For this review, take the finished solid that the model builds, in its own axes (mm). A direction names the side the tool comes from. Round coordinates to 2 decimals unless told otherwise and drop trailing zeros. Write each loop counter-clockwise with the first axis right and the second up, starting at its lowest first coordinate (ties: lowest second). Pieces come first, ordered by that corner, then holes. Notation, with made-up numbers: (3.25, -34.75) -> (45.25, -34.75) arc R29 cw to (45.25, 2.25) -> close; hole circle Ø5 at (-10.5, 14). An arc over 180 degrees is marked (long way). Answer in a Markdown table with one row per item.
Autodesk Inventor part; units mm, degrees
ref_plane "YZ Plane" through (0, 0, 0) normal (1, 0, 0) x (0, 1, 0)
ref_plane "XZ Plane" through (0, 0, 0) normal (0, 1, 0) x (-1, 0, 0)
ref_plane "XY Plane" through (0, 0, 0) normal (0, 0, 1) x (1, 0, 0)
sketch "Esquisse1" plane through (0, 0, 0) normal (0, 0, 1) x (1, 0, 0)
  circle A0 centre (0, 0) radius 2
  line L0 (0, 0) -> (46.5696, 0) construction
  line L1 (0, 0) -> (27.5772, 27.5772) construction
  circle A1 centre (27.5772, 27.5772) radius 2
  line L2 (27.5772, 27.5772) -> (55.1548, 4.4368) construction
  line L3 (27.5772, 27.5772) -> (45.4581, 27.5772) construction
  line L4 (0, 0) -> (0, -8) construction
  line L5 (0, 0) -> (-5.6569, 5.6569) construction
  line L6 (27.5772, 27.5772) -> (27.5772, 35.5772) construction
  line L7 (27.5772, 27.5772) -> (36.2548, 37.9188) construction
  line L8 (36.2548, 37.9188) -> (41.2341, 33.7406) construction
  line L9 (41.2341, 33.7406) -> (47.3624, 28.5983) construction
  line L10 (47.3624, 28.5983) -> (53.4908, 23.456) construction
  line L11 (53.4908, 23.456) -> (59.6192, 18.3137) construction
  line L12 (55.1548, 4.4368) -> (60.2971, 10.5652) construction
  circle A2 centre (41.2341, 33.7406) radius 1 construction
  circle A3 centre (47.3624, 28.5983) radius 1
  circle A4 centre (53.4908, 23.456) radius 1
  circle A5 centre (59.6192, 18.3137) radius 1
  circle A6 centre (60.2971, 10.5652) radius 1
  line L13 (59.6192, 18.3137) -> (67.6192, 18.3137) construction
  line L14 (67.6192, 35.5772) -> (67.6192, -8)
  line L15 (67.6192, -8) -> (-17.1163, -8)
  line L16 (-17.1163, -8) -> (19.4493, 35.5772)
  line L17 (19.4493, 35.5772) -> (67.6192, 35.5772)
  circle A7 centre (23.8788, 13.0574) radius 1 construction
  circle A8 centre (30.0072, 7.9151) radius 1
  circle A9 centre (36.1355, 2.7728) radius 1
  circle A10 centre (42.2639, -2.3695) radius 1
  circle A11 centre (50.0125, -1.6915) radius 1
  line L18 (0, 0) -> (25, 0) construction
  circle A12 centre (25, 0) radius 2
  dimension "d0" = 4
  dimension "d1" = 39
  dimension "d2" = 45
  dimension "d3" = 36
  dimension "d4" = 40
  dimension "d5" = 8
  dimension "d6" = 8
  dimension "d7" = 8
  dimension "d8" = 13.5
  dimension "d9" = 6.5
  dimension "d10" = 8
  dimension "d11" = 8
  dimension "d12" = 8
  dimension "d13" = 8
  dimension "d14" = 2
  dimension "d15" = 8
  dimension "d16" = 25
extrude "Extrusion1" add sketch "Esquisse1" along normal blind 12
sketch "Esquisse2" plane through (0, 0, 0) normal (0, 0, -1) x (-1, 0, 0)
  circle A0 centre (-27.5772, 27.5772) radius 2
  circle A1 centre (0, 0) radius 2
  line L0 (17.1163, -8) -> (-19.4493, 35.5772)
  line L1 (-19.4493, 35.5772) -> (-67.6192, 35.5772)
  circle A2 centre (-27.5772, 27.5772) radius 12 construction
  line L2 (-39.5772, 35.5772) -> (-39.5772, 27.5772)
  line L3 (4.7219, 6.771) -> (-30.5997, 15.964)
  arc A3 (-39.5772, 27.5772) -> (-30.5997, 15.964) centre (-27.5772, 27.5772) ccw
  line L4 (-67.6192, -8) -> (17.1163, -8)
  line L5 (0, 0) -> (0, 8) construction
  dimension "d19" = 24
  dimension "d42" = 8
extrude "Extrusion2" cut sketch "Esquisse2" against normal blind 7 contours L3 A3 L2 L1 L0
sketch "Esquisse3" plane through (0, 0, 7) normal (0, 0, -1) x (-1, 0, 0)
  circle A0 centre (-27.5772, 27.5772) radius 2
  arc A1 (-39.5772, 27.5772) -> (-30.5997, 15.964) centre (-27.5772, 27.5772) ccw
  circle A2 centre (-27.5772, 27.5772) radius 4
  point P0 (0, 0)
  dimension "d24" = 8
extrude "Extrusion3" cut sketch "Esquisse3" against normal through all
fillet "Congé1" radius 8 1 edges at (-17.1163, -8, 6)
fillet "Congé2" radius 10 1 edges at (19.4493, 35.5772, 9.5)
fillet "Congé5" radius 8 1 edges at (39.5772, 35.5772, 3.5)
chamfer "Chanfrein1" distance 15 angle 45 1 edges at (67.6192, 35.5772, 6)
chamfer "Chanfrein2" distance 15 angle 45 1 edges at (67.6192, -8, 6)
fillet "Congé6" radius 10 1 edges at (67.6192, 20.5772, 6)
fillet "Congé7" radius 10 1 edges at (52.6192, 35.5772, 6)
fillet "Congé8" radius 10 1 edges at (67.6192, 7, 6)
fillet "Congé9" radius 10 1 edges at (52.6192, -8, 6)
properties part number "joint1left+ax12imprint_v3"
1) Consider section C-C on x = 25. State the section outline as (y, z) points.
Solved:
| item | result |
|---|---|
| outline | (-8, 0) -> (-2, 0) -> (-2, 12) -> (-8, 12) -> close; (2, 0) -> (14.51, 0) -> (14.51, 7) -> (24.52, 7) -> (24.52, 12) -> (2, 12) -> close; (30.64, 7) -> (35.58, 7) -> (35.58, 12) -> (30.64, 12) -> close |
2) Consider section A-A on x = 1. State the section outline as (y, z) points, then the cut area to 3 significant figures.
Solved:
| item | result |
|---|---|
| outline | (-8, 0) -> (-1.73, 0) -> (-1.73, 12) -> (-8, 12) -> close; (1.73, 0) -> (8.26, 0) -> (8.26, 7) -> (13.59, 7) -> (13.59, 12) -> (1.73, 12) -> close |
| area | 180 mm² |
3) Consider section B-B on z = 10. State how many separate pieces and enclosed holes the cut face has, then the cut area to 3 significant figures.
Solved:
| item | result |
|---|---|
| separate pieces | 1 |
| enclosed holes | 11 |
| area | 2,490 mm² |
4) For faces 1 (the flat face through (60.06, -0.56, 5.92)), 2 (the flat face through (22, 21, 7)), list the 3-axis set-ups (+Z, -Z, +X, -X, +Y, -Y) from which the entire face can be reached by the end or side of a thin tool; tool diameter is ignored.
Solved:
| item | result |
|---|---|
| face 1 | +Z, -Z, +X, -Y |
| face 2 | -Z, -X, +Y |
5) For line 1 (X direction, y = -1, z = 9.5); line 2 (X direction, y = 1, z = 6.25); line 3 (X direction, y = -1.5, z = 4.25), list the stretches that pass through material, from the lowest coordinate up. Write a range as [from, to].
Solved:
| item | result |
|---|---|
| line 1 | [-7.9, -1.73], [1.73, 23.27], [26.73, 49.29], [50.73, 59.62] |
| line 2 | [-7.9, -1.73], [1.73, 23.27], [26.73, 61.62] |
| line 3 | [-7.82, -1.32], [1.32, 23.68], [26.32, 41.77], [42.76, 49.03], [50.99, 59.12] |
6) Clearance check with flat-ended pins moving along their axes: pin 1 Ø2.5 at (x, y) = (36.14, 2.77) entering from +Z; pin 2 Ø1.5 at (y, z) = (9, 10) entering from +X. State where each tip first meets the part, or that it passes through.
Solved:
| item | result |
|---|---|
| pin 1 | z = 12 |
| pin 2 | x = 67.52 |
